Part print with two shaded views. Sizes in mm from the minimum x, y, z corner. A direction names the side the tool comes from. Round coordinates to 2 decimals unless told otherwise and drop trailing zeros. Order: outer loops, then holes, each group sorted by start corner. A loop starts at its lowest first (then second) coordinate and runs counter-clockwise, first axis right, second up. Notation, with made-up numbers: (19.25, 32) -> (74.25, 32) arc R18 cw to (74.25, 38) -> close; hole circle Ø4 at (4, -19). An arc over 180 degrees is marked (long way). Answer as a JSON object with one key per item and string values.
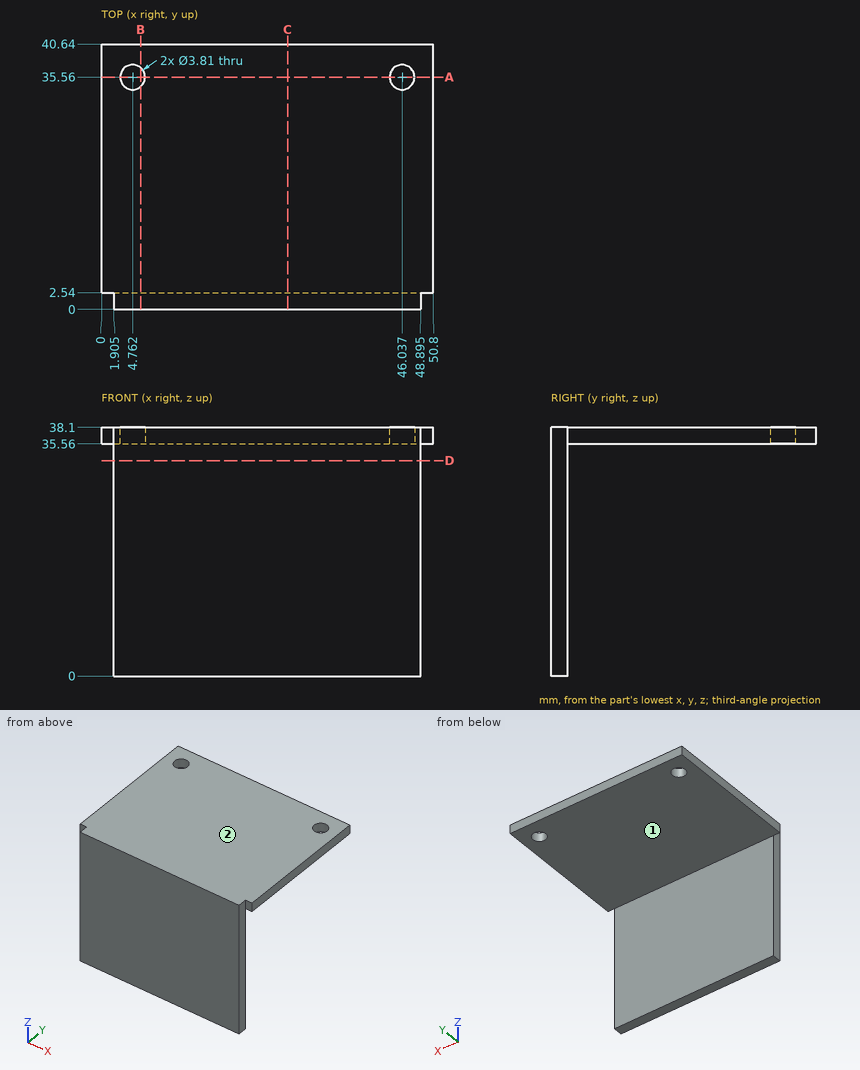
1) Cut at C-C, the plane x = 28.5. Give the cut face in (y, z).
Checked values:
{"outline": "(0, 0) -> (2.54, 0) -> (2.54, 35.56) -> (40.64, 35.56) -> (40.64, 38.1) -> (0, 38.1) -> close"}
2) Probe L1, parallel to X at y = 35, z = 36; L2, parallel to Z at x = 11.5, y = 37.5; L3, parallel to Y at x = 18, z = 25.5. List the from-to ranges inside material, lowest first. Write a range as from..to.
Checked values:
{"L1": "x = 0..2.94, 6.58..44.22, 47.86..50.8", "L2": "z = 35.56..38.1", "L3": "y = 0..2.54"}
3) Cut at A-A, the plane y = 35.56. Give the cut face in (x, z).
Checked values:
{"outline": "(0, 35.56) -> (2.86, 35.56) -> (2.86, 38.1) -> (0, 38.1) -> close; (6.67, 35.56) -> (44.13, 35.56) -> (44.13, 38.1) -> (6.67, 38.1) -> close; (47.94, 35.56) -> (50.8, 35.56) -> (50.8, 38.1) -> (47.94, 38.1) -> close"}
4) Flat gauge pins, fed straight in: pin 1 Ø3 at (y, z) = (1.5, 28.5) entering from -X (1 decimal); pin 2 Ø5 at (x, z) = (29, 15) entering from +Y; pin 3 Ø6 at (x, y) = (4.76, 35.56) entering from -Z; pin 4 Ø3.5 at (x, y) = (46.04, 35.56) entering from +Z. Where does each tip first touch, or does it go through?
Checked values:
{"pin 1": "stops at x = 1.9", "pin 2": "stops at y = 2.54", "pin 3": "stops at z = 35.56", "pin 4": "passes through"}
5) Which spindle directions (+Z, -Z, +X, -X, +Y, -Y) get a long thin tool onto all of the face, cutting with end or side? Do the marked faces 1 and 2. Say none if no direction does.
Checked values:
{"face 1": "-Z, +X, -X, +Y", "face 2": "+Z, +X, -X, +Y, -Y"}
6) Cut at D-D, the plane z = 33. Give the cut face in (x, y) (1 decimal).
Checked values:
{"outline": "(1.9, 0) -> (48.9, 0) -> (48.9, 2.5) -> (1.9, 2.5) -> close"}
7) Cut at B-B, the plane x = 6. Give the cut face in (y, z).
Checked values:
{"outline": "(0, 0) -> (2.54, 0) -> (2.54, 35.56) -> (34.11, 35.56) -> (34.11, 38.1) -> (0, 38.1) -> close; (37.01, 35.56) -> (40.64, 35.56) -> (40.64, 38.1) -> (37.01, 38.1) -> close"}
